Study the drawing (mm; zero at the part's minimum x, y, z) and answer. Coordinates: 2 decimals unless noted, no trailing zeros. Loops run counter-clockwise (first coordinate to the right, second up) from the corner with the lowest first, then second, coordinate; pieces in that order, holes last. Notation, with made-up numbers: (78, -8.75) -> (90, -8.75) arc R23 ccw to (90, 11.25) -> close; hole circle Ø4 at (25.5, -3.5). An arc over 180 degrees is marked (long way). Answer as a JSON object with one key per item and string values. Group by question number.
Q1. Straight lines are drawn through the part: line 1 along X through (y, z) = (8.75, 10); line 2 along Z through (x, y) = (9.75, 27.5); line 3 along X through (y, z) = (6.5, 9.25). For each, find the intervals that lie inside material, in ascending order. Write a range as [from, to].
Q2. Each of these flat-tipped pins is pushed along its axis until it touches: P1, Ø3, axis at x = 9, z = 10, coming from the +Y side; P2, Ø6, axis at x = 3, y = 26, coming from the +Z side; P3, Ø2, axis at x = 2.5, y = 22, coming from the -Z side. Where does it stop, or does it pass through?
Q3. The part is cut by section B-B on y = 5. Write down the section's boundary in (x, z).
Q4. Determine the mould class of the marked faces 1, 2 and 3 for opening direction Z: released by +Z, released by -Z, zero draft, split by the parting line, or undercut.
Q5. The part is cut by section A-A on z = 10. Write down the section's boundary in (x, y).
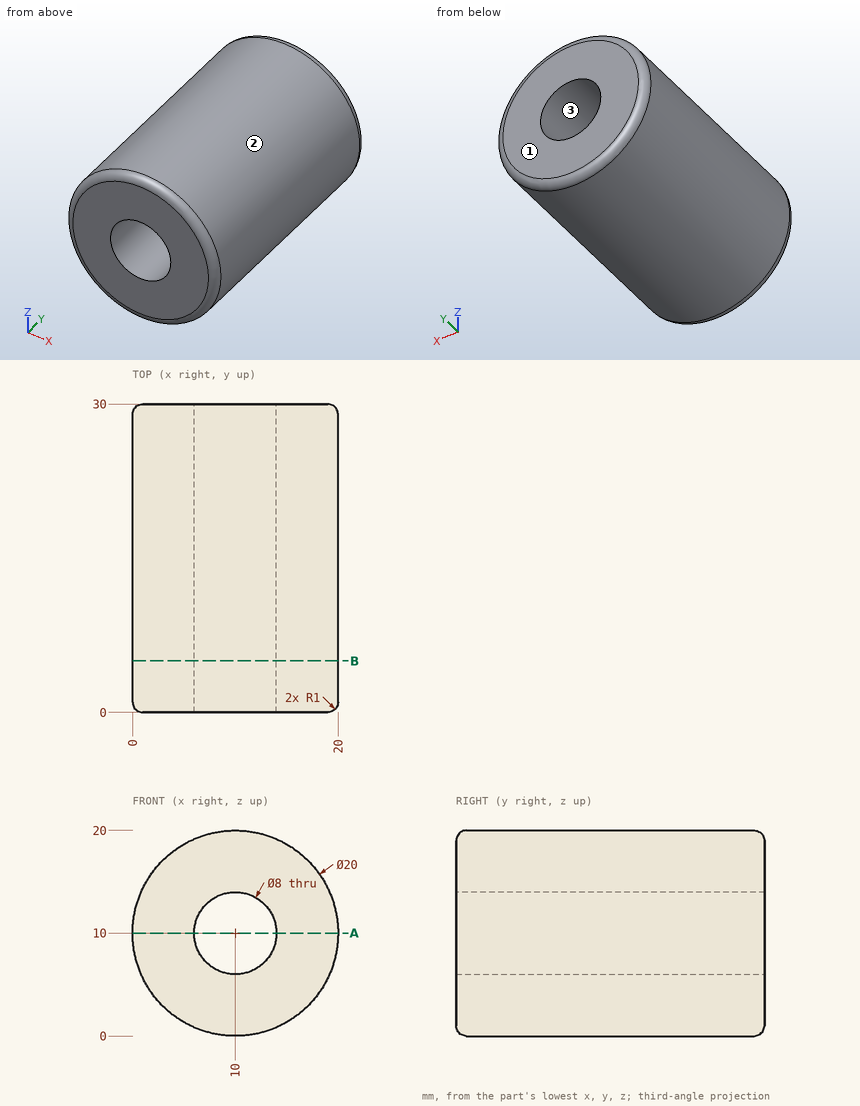
Final values:
{
 "1": {"line 1": "x = [0, 6], [14, 20]", "line 2": "z = [0, 6.01], [13.99, 20]", "line 3": "x = [0.03, 6.07], [13.93, 19.97]"},
 "2": {"P1": "passes through", "P2": "stops at z = 19.17", "P3": "stops at z = 2.4"},
 "3": {"outline": "circle Ø20 at (10, 10); hole circle Ø8 at (10, 10)"},
 "4": {"face 1": "zero draft", "face 2": "split by the parting line", "face 3": "undercut"},
 "5": {"outline": "(0, 1) arc R1 ccw to (1, 0) -> (6, 0) -> (6, 30) -> (1, 30) arc R1 ccw to (0, 29) -> close; (14, 0) -> (19, 0) arc R1 ccw to (20, 1) -> (20, 29) arc R1 ccw to (19, 30) -> (14, 30) -> close"}
}
